```python
from build123d import *

# Parameters (mm, degrees)
SKETCH1_W                     = 20
SKETCH1_H                     = 45
BOSS_EXTRUDE1_DEPTH           = 2
M5_CLEARANCE_HOLE1_AT_2_COUNT = 2
M5_CLEARANCE_HOLE1_AT_2_PITCH = 22


with BuildPart() as part:
    # Sketch1 → Boss-Extrude1 (new body)
    with BuildSketch(Plane.XY):
        with Locations((10, 22.5)):
            Rectangle(SKETCH1_W, SKETCH1_H)
    extrude(amount=BOSS_EXTRUDE1_DEPTH)

    # Sketch3 → M5 Clearance Hole1 (revolve, cut)
    with BuildSketch(Plane(origin=(10, 30, 2), x_dir=(0, -1, 0), z_dir=(1, 0, 0))):
        Polygon((0, 0), (0, 2), (2.75, 2), (2.75, 0.025), (2.775, 0), align=None)
    m5_clearance_hole1 = revolve(axis=Axis((10, 30, 8.35), (0, 0, -1)), mode=Mode.SUBTRACT)

    # M5 Clearance Hole1 at 2: M5 Clearance Hole1 ×2
    with Locations(*[(0, -i * M5_CLEARANCE_HOLE1_AT_2_PITCH, 0) for i in range(1, M5_CLEARANCE_HOLE1_AT_2_COUNT)]):
        add(m5_clearance_hole1, mode=Mode.SUBTRACT)


solid = part.part
```
Design review of the part built by this model. Coordinates are the model's own, in mm. Coordinates: 2 decimals unless noted, no trailing zeros. Loops run counter-clockwise (first coordinate to the right, second up) from the corner with the lowest first, then second, coordinate; pieces in that order, holes last. Notation, with made-up numbers: (69.5, 26) -> (106.5, 26) arc R12 ccw to (106.5, 39) -> close; hole circle Ø8 at (-27.75, -26). An arc over 180 degrees is marked (long way). Answer as a JSON object with one key per item and string values.
Q1. Take a section at B-B on x = 10. Give the boundary of the cut face in (y, z) (3 decimals), plus the area to 3 significant figures.
Answer block:
{"outline": "(0, 0) -> (5.25, 0) -> (5.25, 1.975) -> (5.225, 2) -> (0, 2) -> close; (10.75, 0) -> (27.25, 0) -> (27.25, 1.975) -> (27.225, 2) -> (10.775, 2) -> (10.75, 1.975) -> close; (32.75, 0) -> (45, 0) -> (45, 2) -> (32.775, 2) -> (32.75, 1.975) -> close", "area": "68.0 mm^2"}
Q2. The part is to be moulded in two halves that separate along X. For faces 1 (the flat face through (10, 0, 1)), 2 (the cylindrical face through (11.05, 5.46, 1)), 3 (the flat face through (0, 22, 1)), 4 (the cylindrical face through (9.879, 32.747, 1.001)), say which applies: +X half, -X half, draft (parallel to the pull), parting line (faces both ways), or undercut.
Answer block:
{"face 1": "draft", "face 2": "undercut", "face 3": "-X half", "face 4": "undercut"}
Q3. To check wall thickness, follow L1, parallel to Y at x = 10, z = 1.2; L2, parallel to X at y = 8, z = 1.25; L3, parallel to Y at x = 9.25, z = 0.6. State the ranges of each line that lie inside material, in increasing order.
Answer block:
{"L1": "y = 0 to 5.25, 10.75 to 27.25, 32.75 to 45", "L2": "x = 0 to 7.25, 12.75 to 20", "L3": "y = 0 to 5.35, 10.65 to 27.35, 32.65 to 45"}
Q4. Take a section at C-C on z = 0.7. Give the boundary of the cut face in (x, y).
Answer block:
{"outline": "(0, 0) -> (20, 0) -> (20, 45) -> (0, 45) -> close; hole circle Ø5.5 at (10, 8); hole circle Ø5.5 at (10, 30)"}
Q5. Take a section at A-A on y = 30. Give the boundary of the cut face in (x, z) (3 decimals).
Answer block:
{"outline": "(0, 0) -> (7.25, 0) -> (7.25, 1.975) -> (7.225, 2) -> (0, 2) -> close; (12.75, 0) -> (20, 0) -> (20, 2) -> (12.775, 2) -> (12.75, 1.975) -> close"}
